Design review of the part built by this model. Coordinates are the model's own, in mm. Face numbers are marked on the shaded views. A direction names the side the tool comes from. Coordinates: 2 decimals unless noted, no trailing zeros. Loops run counter-clockwise (first coordinate to the right, second up) from the corner with the lowest first, then second, coordinate; pieces in that order, holes last.
Q1. Draft analysis for pull direction X (two halves, no side actions). For the marked faces 1, 2 and 3, state which applies: released by +X, released by -X, zero draft, split by the parting line, or undercut.
Q2. Machinability: for the marked faces 4, 5, 6, 7 and 8, which of the approach directions +Z, -Z, +X, -X, +Y, -Y give a long, thin tool a straight path to every point of the face, cutting with its end or side? Answer none if there is none.
Q3. Add section B-B on x = 38.1. Give the boundary of the cut face in (y, z).
Q4. Add section A-A on x = 6. Give the boundary of the cut face in (y, z), and give its area (3 significant figures).
Q5. Wall thickness on probe 1 along X at (y, z) = (52, -7); probe 2 along Z at (x, y) = (4.5, 58); probe 3 along Z at (x, y) = (-10, 53.5): over which ranges is each line inside the solid? List them lowest first.
Q6. Add section C-C on x = 57.5. Give the boundary of the cut face in (y, z), and give its area (3 significant figures).
Q7. For P1, Ø12.5, axis at y = 142, z = -5.5, coming from the +X side; P2, Ø0.7, axis at x = -1.5, z = 20.5, coming from the +Y side; P3, Ø12.5, axis at y = 145, z = 5, coming from the -X side; P4, Ø1, axis at x = 4.5, z = -19, coming from the -Y side, all flat-tipped, find the tip position at first contact; note any pin that passes through.
Q8. Add section D-D on y = 118. Give the boundary of the cut face in (x, z), and give its area (3 significant figures).
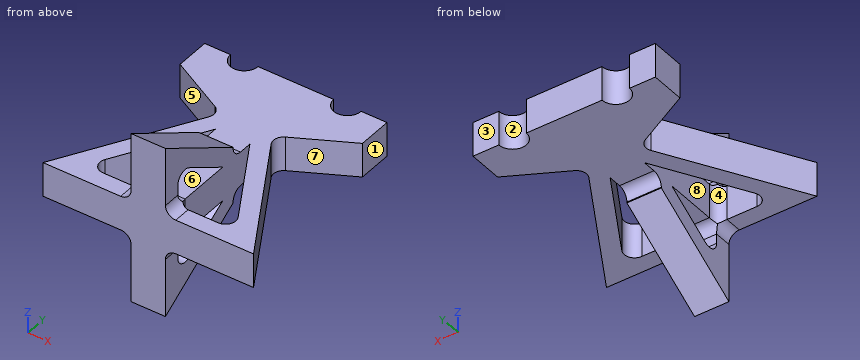
```python
from build123d import *

# Parameters (mm, degrees)
BOSS_EXTRUDE1_DEPTH      = 12.7
BOSS_EXTRUDE1_DEPTH_BACK = 12.7
BOSS_EXTRUDE2_DEPTH      = 12.7
BOSS_EXTRUDE2_DEPTH_BACK = 12.7
FILLET1_R                = 7.62
FILLET2_R                = 7.62
FILLET3_R                = 7.62


with BuildPart() as part:
    # Sketch1 → Boss-Extrude1 (new, two sides: drawn at the far end of the back side and taken through both)
    with BuildSketch(Plane.XY.offset(-BOSS_EXTRUDE1_DEPTH_BACK)):
        with BuildLine():
            Line((27.94, 152.4), (-27.94, 152.4))
            ThreePointArc((-27.94, 152.4), (-38.1, 142.24), (-48.26, 152.4))
            Line((-48.26, 152.4), (-67.31, 152.4))
            Line((-67.31, 152.4), (-67.31, 127))
            Line((-67.31, 127), (-19.05, 101.6))
            Line((-19.05, 101.6), (-77.70878735, 0))
            Line((-77.70878735, 0), (77.70878735, 0))
            Line((77.70878735, 0), (19.05, 101.6))
            Line((19.05, 101.6), (67.31, 127))
            Line((67.31, 127), (67.31, 152.4))
            Line((67.31, 152.4), (48.26, 152.4))
            ThreePointArc((48.26, 152.4), (38.1, 142.24), (27.94, 152.4))
        make_face()
        Polygon((-55.711742094, 12.7), (-12.7, 12.7), (-12.7, 87.198522628), align=None, mode=Mode.SUBTRACT)
        Polygon((12.7, 87.198522628), (12.7, 12.7), (55.711742094, 12.7), align=None, mode=Mode.SUBTRACT)
    extrude(amount=BOSS_EXTRUDE1_DEPTH + BOSS_EXTRUDE1_DEPTH_BACK)

    # Sketch2 → Boss-Extrude2 (add, two sides: drawn at the far end of the back side and taken through both)
    with BuildSketch(Plane(origin=(0, 0, 0), x_dir=(0, 0, -1), z_dir=(1, 0, 0)).offset(-BOSS_EXTRUDE2_DEPTH_BACK)):
        Polygon((20.992545931, 69.85), (63.5, 0), (-63.5, 0), (-20.992545931, 69.85), align=None)
        Polygon((12.7, 59.046917663), (40.904573712, 12.7), (12.7, 12.7), align=None, mode=Mode.SUBTRACT)
        Polygon((-12.7, 59.046917663), (-12.7, 12.7), (-40.904573712, 12.7), align=None, mode=Mode.SUBTRACT)
    extrude(amount=BOSS_EXTRUDE2_DEPTH + BOSS_EXTRUDE2_DEPTH_BACK)

    # Fillet1
    fillet1_edges = [part.edges().sort_by_distance(p)[0] for p in [
        (0, 69.85, -12.7),
        (0, 69.85, 12.7),
    ]]
    fillet(fillet1_edges, radius=FILLET1_R)

    # Fillet2
    # the kernel refuses this fillet: 7.62 mm, written as the material it adds along each edge
    with BuildSketch(Plane(origin=(12.7, 12.7, -12.7), x_dir=(0, 0, -1), z_dir=(0, -1, 0)), Plane(origin=(12.7, 12.7, 12.7), x_dir=(1, 0, 0), z_dir=(0, -1, 0))) as fillet2_piece_1:
        with BuildLine():
            CenterArc((FILLET2_R, FILLET2_R), FILLET2_R, 180, 90)
            Line((0, FILLET2_R), (0, 0))
            Line((0, 0), (FILLET2_R, 0))
        make_face()
    extrude(amount=12.7)
    with BuildSketch(Plane(origin=(-12.7, 12.7, -12.7), x_dir=(0, 0, -1), z_dir=(0, -1, 0)), Plane(origin=(-12.7, 12.7, 12.7), x_dir=(-1, 0, 0), z_dir=(0, -1, 0))) as fillet2_piece_2:
        with BuildLine():
            CenterArc((FILLET2_R, -FILLET2_R), FILLET2_R, 90, 90)
            Line((0, -FILLET2_R), (0, 0))
            Line((0, 0), (FILLET2_R, 0))
        make_face()
    extrude(amount=12.7)
    with BuildSketch(Plane(origin=(12.7, 12.7, -40.904573712), x_dir=(0, 0, 1), z_dir=(-1, 0, 0)), Plane(origin=(12.7, 12.7, 40.904573712), x_dir=(0, 0.8542525273339658, -0.5198582687074736), z_dir=(-1, 0, 0))) as fillet2_piece_3:
        with BuildLine():
            CenterArc((FILLET2_R * 1.77916742424, FILLET2_R), FILLET2_R, 148.677255076, 121.322744924)
            Line((FILLET2_R * 0.924914896906, FILLET2_R * 1.51985826871), (0, 0))
            Line((0, 0), (FILLET2_R * 1.77916742424, 0))
        make_face()
    extrude(amount=25.4)
    with BuildSketch(Plane(origin=(19.05, 101.6, -12.7), x_dir=(0.4999999999999972, -0.8660254037844403, 0), z_dir=(0, 0, 1))) as fillet2_piece_4:
        with BuildLine():
            CenterArc((FILLET2_R * 1.03990652475, FILLET2_R), FILLET2_R, 177.758540601, 92.241459399)
            Line((FILLET2_R * 0.0406716474833, FILLET2_R * 1.03911086864), (0, 0))
            Line((0, 0), (FILLET2_R * 1.03990652475, 0))
        make_face()
    extrude(amount=25.4)
    with BuildSketch(Plane(origin=(-19.05, 101.6, -12.7), x_dir=(-0.4999999999999979, -0.8660254037844399, 0), z_dir=(0, 0, 1))) as fillet2_piece_5:
        with BuildLine():
            CenterArc((FILLET2_R * 1.03990652475, -FILLET2_R), FILLET2_R, 90, 92.241459399)
            Line((FILLET2_R * 0.0406716474833, -FILLET2_R * 1.03911086864), (0, 0))
            Line((0, 0), (FILLET2_R * 1.03990652475, 0))
        make_face()
    extrude(amount=25.4)
    with BuildSketch(Plane(origin=(-55.711742094, 12.7, 12.7), x_dir=(0.49999999999999845, 0.8660254037844396, 0), z_dir=(0, 0, -1)), Plane(origin=(55.711742094, 12.7, -12.7), x_dir=(-0.4999999999999981, 0.8660254037844397, 0), z_dir=(0, 0, 1))) as fillet2_piece_6:
        with BuildLine():
            CenterArc((FILLET2_R * 1.73205080757, FILLET2_R), FILLET2_R, 150, 120)
            Line((FILLET2_R * 0.866025403784, FILLET2_R * 1.5), (0, 0))
            Line((0, 0), (FILLET2_R * 1.73205080757, 0))
        make_face()
    extrude(amount=25.4)

    # Fillet3
    # the kernel refuses this fillet: 7.62 mm, written as the material it adds along each edge
    with BuildSketch(Plane(origin=(12.7, 12.7, -12.7), x_dir=(1, 0, 0), z_dir=(0, 0, 1)), Plane(origin=(12.7, 12.7, 12.7), x_dir=(0, 0, 1), z_dir=(-1, 0, 0))) as fillet3_piece_1:
        with BuildLine():
            CenterArc((FILLET3_R, FILLET3_R), FILLET3_R, 180, 90)
            Line((0, FILLET3_R), (0, 0))
            Line((0, 0), (FILLET3_R, 0))
        make_face()
    extrude(amount=25.4)
    with BuildSketch(Plane(origin=(12.7, 12.7, -12.7), x_dir=(0, 0, -1), z_dir=(-1, 0, 0)), Plane(origin=(-12.7, 12.7, -12.7), x_dir=(-1, 0, 0), z_dir=(0, 0, 1))) as fillet3_piece_2:
        with BuildLine():
            CenterArc((FILLET3_R, -FILLET3_R), FILLET3_R, 90, 90)
            Line((0, -FILLET3_R), (0, 0))
            Line((0, 0), (FILLET3_R, 0))
        make_face()
    extrude(amount=25.4)
    with BuildSketch(Plane(origin=(31.75, 12.7, -12.7), x_dir=(0, 0, -1), z_dir=(-1, 0, 0))) as fillet3_piece_3a_section:
        with BuildLine():
            CenterArc((FILLET3_R, -FILLET3_R), FILLET3_R, 90, 90)
            Line((0, -FILLET3_R), (0, 0))
            Line((0, 0), (FILLET3_R, 0))
        make_face()
    fillet3_piece_3a = extrude(amount=44.45, mode=Mode.PRIVATE)
    fillet3_piece_3a = split(fillet3_piece_3a, bisect_by=Plane(origin=(12.7, 14.893212432, -14.893212432), z_dir=(1, 0, 0)), keep=Keep.TOP, mode=Mode.PRIVATE)
    fillet3_piece_3a = fillet3_piece_3a - Plane(origin=(20.32, 14.893212432, -20.32), x_dir=(0, 0, -1), z_dir=(0, 1, 0)) * Cylinder(7.62, 120, mode=Mode.PRIVATE)
    with BuildSketch(Plane(origin=(12.7, 12.7, -31.75), x_dir=(1, 0, 0), z_dir=(0, 0, 1))) as fillet3_piece_3b_section:
        with BuildLine():
            CenterArc((FILLET3_R, FILLET3_R), FILLET3_R, 180, 90)
            Line((0, FILLET3_R), (0, 0))
            Line((0, 0), (FILLET3_R, 0))
        make_face()
    fillet3_piece_3b = extrude(amount=44.45, mode=Mode.PRIVATE)
    fillet3_piece_3b = fillet3_piece_3b - Plane(origin=(20.32, 13.018424072, -20.32), x_dir=(0, 0, -1), z_dir=(0, 1, 0)) * Cylinder(7.62, 120, mode=Mode.PRIVATE)
    fillet3_piece_3b = split(fillet3_piece_3b, bisect_by=Plane(origin=(17.997172091, 13.018424072, -12.7), z_dir=(0, 0, -1)), keep=Keep.TOP, mode=Mode.PRIVATE)
    fillet3_piece_3b = fillet3_piece_3b - Plane(origin=(17.997172091, 20.32, -27.347317939), x_dir=(0, 0, 1), z_dir=(1, 0, 0)) * Cylinder(7.62, 120, mode=Mode.PRIVATE)
    fillet3_piece_3 = fillet3_piece_3a & fillet3_piece_3b
    add(fillet3_piece_3)
    with BuildSketch(Plane(origin=(31.75, 12.7, 12.7), x_dir=(0, 0, 1), z_dir=(-1, 0, 0))) as fillet3_piece_4a_section:
        with BuildLine():
            CenterArc((FILLET3_R, FILLET3_R), FILLET3_R, 180, 90)
            Line((0, FILLET3_R), (0, 0))
            Line((0, 0), (FILLET3_R, 0))
        make_face()
    fillet3_piece_4a = extrude(amount=44.45, mode=Mode.PRIVATE)
    fillet3_piece_4a = fillet3_piece_4a - Plane(origin=(20.32, 14.893212432, 20.32), x_dir=(1, 0, 0), z_dir=(0, 1, 0)) * Cylinder(7.62, 120, mode=Mode.PRIVATE)
    fillet3_piece_4a = split(fillet3_piece_4a, bisect_by=Plane(origin=(12.7, 14.893212432, 14.893212432), z_dir=(1, 0, 0)), keep=Keep.TOP, mode=Mode.PRIVATE)
    with BuildSketch(Plane(origin=(12.7, 12.7, -12.7), x_dir=(1, 0, 0), z_dir=(0, 0, 1))) as fillet3_piece_4b_section:
        with BuildLine():
            CenterArc((FILLET3_R, FILLET3_R), FILLET3_R, 180, 90)
            Line((0, FILLET3_R), (0, 0))
            Line((0, 0), (FILLET3_R, 0))
        make_face()
    fillet3_piece_4b = extrude(amount=44.45, mode=Mode.PRIVATE)
    fillet3_piece_4b = split(fillet3_piece_4b, bisect_by=Plane(origin=(14.346750692, 12.818924561, 12.7), z_dir=(0, 0, 1)), keep=Keep.TOP, mode=Mode.PRIVATE)
    fillet3_piece_4b = fillet3_piece_4b - Plane(origin=(20.32, 12.818924561, 20.32), x_dir=(1, 0, 0), z_dir=(0, 1, 0)) * Cylinder(7.62, 120, mode=Mode.PRIVATE)
    fillet3_piece_4b = fillet3_piece_4b - Plane(origin=(14.346750692, 20.32, 27.347317939), x_dir=(0, 0.8542525273341854, -0.5198582687071128), z_dir=(1, 0, 0)) * Cylinder(7.62, 120, mode=Mode.PRIVATE)
    fillet3_piece_4 = fillet3_piece_4a & fillet3_piece_4b
    add(fillet3_piece_4)
    with BuildSketch(Plane(origin=(-12.7, 12.7, -31.75), x_dir=(-1, 0, 0), z_dir=(0, 0, 1))) as fillet3_piece_5a_section:
        with BuildLine():
            CenterArc((FILLET3_R, -FILLET3_R), FILLET3_R, 90, 90)
            Line((0, -FILLET3_R), (0, 0))
            Line((0, 0), (FILLET3_R, 0))
        make_face()
    fillet3_piece_5a = extrude(amount=44.45, mode=Mode.PRIVATE)
    fillet3_piece_5a = split(fillet3_piece_5a, bisect_by=Plane(origin=(-17.997172063, 13.018423982, -12.7), z_dir=(0, 0, -1)), keep=Keep.TOP, mode=Mode.PRIVATE)
    fillet3_piece_5a = fillet3_piece_5a - Plane(origin=(-20.32, 13.018423982, -20.32), x_dir=(0, 0, -1), z_dir=(0, 1, 0)) * Cylinder(7.62, 120, mode=Mode.PRIVATE)
    fillet3_piece_5a = fillet3_piece_5a - Plane(origin=(-17.997172063, 20.32, -27.347317939), x_dir=(0, 0, 1), z_dir=(1, 0, 0)) * Cylinder(7.62, 120, mode=Mode.PRIVATE)
    with BuildSketch(Plane(origin=(12.7, 12.7, -12.7), x_dir=(0, 0, -1), z_dir=(-1, 0, 0))) as fillet3_piece_5b_section:
        with BuildLine():
            CenterArc((FILLET3_R, -FILLET3_R), FILLET3_R, 90, 90)
            Line((0, -FILLET3_R), (0, 0))
            Line((0, 0), (FILLET3_R, 0))
        make_face()
    fillet3_piece_5b = extrude(amount=44.45, mode=Mode.PRIVATE)
    fillet3_piece_5b = fillet3_piece_5b - Plane(origin=(-20.32, 20.265363421, -20.32), x_dir=(0, 0, -1), z_dir=(0, 1, 0)) * Cylinder(7.62, 120, mode=Mode.PRIVATE)
    fillet3_piece_5b = split(fillet3_piece_5b, bisect_by=Plane(origin=(-12.7, 20.265363421, -12.6238), z_dir=(-1, 0, 0)), keep=Keep.TOP, mode=Mode.PRIVATE)
    fillet3_piece_5 = fillet3_piece_5a & fillet3_piece_5b
    add(fillet3_piece_5)
    with BuildSketch(Plane(origin=(-12.7, 12.7, -12.7), x_dir=(-1, 0, 0), z_dir=(0, 0, 1))) as fillet3_piece_6a_section:
        with BuildLine():
            CenterArc((FILLET3_R, -FILLET3_R), FILLET3_R, 90, 90)
            Line((0, -FILLET3_R), (0, 0))
            Line((0, 0), (FILLET3_R, 0))
        make_face()
    fillet3_piece_6a = extrude(amount=44.45, mode=Mode.PRIVATE)
    fillet3_piece_6a = fillet3_piece_6a - Plane(origin=(-20.32, 16.148179969, 20.32), x_dir=(-1, 0, 0), z_dir=(0, 1, 0)) * Cylinder(7.62, 120, mode=Mode.PRIVATE)
    fillet3_piece_6a = split(fillet3_piece_6a, bisect_by=Plane(origin=(-12.657850187, 16.148179969, 12.7), z_dir=(0, 0, 1)), keep=Keep.TOP, mode=Mode.PRIVATE)
    fillet3_piece_6a = fillet3_piece_6a - Plane(origin=(-12.657850187, 20.32, 27.347317939), x_dir=(0, 0.8542525273341854, -0.5198582687071128), z_dir=(1, 0, 0)) * Cylinder(7.62, 120, mode=Mode.PRIVATE)
    with BuildSketch(Plane(origin=(12.7, 12.7, 12.7), x_dir=(0, 0, 1), z_dir=(-1, 0, 0))) as fillet3_piece_6b_section:
        with BuildLine():
            CenterArc((FILLET3_R, FILLET3_R), FILLET3_R, 180, 90)
            Line((0, FILLET3_R), (0, 0))
            Line((0, 0), (FILLET3_R, 0))
        make_face()
    fillet3_piece_6b = extrude(amount=44.45, mode=Mode.PRIVATE)
    fillet3_piece_6b = split(fillet3_piece_6b, bisect_by=Plane(origin=(-12.7, 20.265363421, 12.6238), z_dir=(-1, 0, 0)), keep=Keep.TOP, mode=Mode.PRIVATE)
    fillet3_piece_6b = fillet3_piece_6b - Plane(origin=(-20.32, 20.265363421, 20.32), x_dir=(-1, 0, 0), z_dir=(0, 1, 0)) * Cylinder(7.62, 120, mode=Mode.PRIVATE)
    fillet3_piece_6 = fillet3_piece_6a & fillet3_piece_6b
    add(fillet3_piece_6)


solid = part.part
```
Entries:
1. face 1: released by +X
1. face 2: undercut
1. face 3: zero draft
2. face 4: +Z, -Z
2. face 5: +Z, -Z, -X
2. face 6: +X, -X
2. face 7: +Z, -Z, +X
2. face 8: none
3. outline: (0, -12.7) - (12.7, -12.7) - (12.7, 12.7) - (0, 12.7) - close; (43.2, -12.7) - (68.6, -12.7) - (68.6, 12.7) - (43.2, 12.7) - close; (111.63, -12.7) - (142.24, -12.7) - (142.24, 12.7) - (111.63, 12.7) - close
4. outline: (0, -63.5) - (69.85, -20.99) - (69.85, -20.32) arc R7.62 cw to (77.47, -12.7) - (152.4, -12.7) - (152.4, 12.7) - (77.47, 12.7) arc R7.62 cw to (69.85, 20.32) - (69.85, 20.99) - (0, 63.5) - close; hole (12.7, -27.35) arc R7.62 ccw to (24.28, -33.86) - (59.05, -12.7) - (20.32, -12.7) arc R7.62 ccw to (12.7, -20.32) - close; hole (12.7, 20.32) arc R7.62 ccw to (20.32, 12.7) - (59.05, 12.7) - (24.28, 33.86) arc R7.62 ccw to (12.7, 27.35) - close
4. area: 6,820 mm2
5. probe 1: x = -47.69 to -33.02, -12.7 to 12.7, 33.02 to 47.69
5. probe 2: z = -28.2 to -13.34, -12.7 to 12.7, 13.34 to 28.2
5. probe 3: z = -30.94 to -16.08, -12.7 to 12.7, 16.08 to 30.94
6. outline: (0, -12.7) - (35, -12.7) - (35, 12.7) - (0, 12.7) - close; (121.84, -12.7) - (152.4, -12.7) - (152.4, 12.7) - (121.84, 12.7) - close
6. area: 1,670 mm2
7. P1: stops at x = 67.31
7. P2: stops at y = 69.85
7. P3: stops at x = -67.31
7. P4: stops at y = 0
8. outline: (-50.21, -12.7) - (50.21, -12.7) - (50.21, 12.7) - (-50.21, 12.7) - close
8. area: 2,550 mm2
